Autodesk Fusion 360 part; units mm, degrees
sketch "Sketch1" plane through (0, 0, 0) normal (0, 0, 1) x (1, 0, 0) in component "Component"
  line L0 (-13, 0) -> (-13, 6.5)
  line L1 (-13, 0) -> (-13, -6.5)
  line L2 (-13, -6.5) -> (13, -6.5)
  line L3 (13, -6.5) -> (13, 6.5)
  line L4 (13, 6.5) -> (-13, 6.5)
  circle A0 centre (0, 0) radius 3
  line L5 (0, 0) -> (9.75, 0)
  line L6 (0, 0) -> (-9.75, 0)
  circle A1 centre (-9.75, 0) radius 3
  circle A2 centre (9.75, 0) radius 3
  line L7 (13, -6.5) -> (14, -6.5)
  line L8 (14, -6.5) -> (14, 6.5)
  line L9 (14, 6.5) -> (13, 6.5)
  line L10 (-13, 6.5) -> (-14, 6.5)
  line L11 (-14, 6.5) -> (-14, -6.5)
  line L12 (-14, -6.5) -> (-13, -6.5)
  dimension "d2" = 13
  dimension "d3" = 6.5
  dimension "d4" = 6.5
  dimension "d5" = 13
  dimension "d6" = 9.75
  dimension "d7" = 9.75
  dimension "d8" = 6
  dimension "d9" = 6
  dimension "d10" = 13
  dimension "d11" = 13
extrude "Extrude1" add sketch "Sketch1" along normal blind 2.5 in component "Component"
component "Component" placed x (1, 0, 0) y (0, 1, 0) z (0, 0, 1) at (0, 0, 0)
Work out the finished part from the listing and answer in its coordinate system (mm). Coordinates: 2 decimals unless noted, no trailing zeros. Write each loop counter-clockwise with the first axis right and the second up, starting at its lowest first coordinate (ties: lowest second). Pieces come first, ordered by that corner, then holes. Notation, with made-up numbers: (50.25, 1.5) - (98.25, 1.5) arc R24 ccw to (98.25, 20.5) - close; hole circle Ø5 at (74, 6). An arc over 180 degrees is marked (long way). One line per question, with ' | ' between items.
1) Find section A-A, the plane y = 0. Determine the outline of the cut face in (x, z), and give its area (3 significant figures).
Checks:
outline: (-14, 0) - (-12.75, 0) - (-12.75, 2.5) - (-14, 2.5) - close; (-6.75, 0) - (-3, 0) - (-3, 2.5) - (-6.75, 2.5) - close; (3, 0) - (6.75, 0) - (6.75, 2.5) - (3, 2.5) - close; (12.75, 0) - (14, 0) - (14, 2.5) - (12.75, 2.5) - close | area: 25.0 mm2
2) Consider probe 1 along X at (y, z) = (2, 0.85); probe 2 along Y at (x, z) = (-9.75, 0.6); probe 3 along X at (y, z) = (1.5, 1.3). Determine where each line is inside the solid, lowest interval first. Write a range as [from, to].
Checks:
probe 1: [-14, -11.99], [-7.51, -2.24], [2.24, 7.51], [11.99, 14] | probe 2: [-6.5, -3], [3, 6.5] | probe 3: [-14, -12.35], [-7.15, -2.6], [2.6, 7.15], [12.35, 14]
3) Find section C-C, the plane z = 1.05. Determine the outline of the cut face in (x, y), and give its area (3 significant figures).
Checks:
outline: (-14, -6.5) - (14, -6.5) - (14, 6.5) - (-14, 6.5) - close; hole circle Ø6 at (-9.75, 0); hole circle Ø6 at (0, 0); hole circle Ø6 at (9.75, 0) | area: 279 mm2
4) The mould has two halves that part along X. Classify faces 1 (the face through (14, 0, 1)), 2 (the face through (-12.131, 1.825, 1.232)), 3 (the face through (0, -6.5, 1)): +X half, -X half, draft (parallel to the pull), parting line (faces both ways), or undercut.
Checks:
face 1: +X half | face 2: undercut | face 3: draft
5) Find section D-D, the plane x = -11. Determine the outline of the cut face in (y, z), and give its area (3 significant figures).
Checks:
outline: (-6.5, 0) - (-2.73, 0) - (-2.73, 2.5) - (-6.5, 2.5) - close; (2.73, 0) - (6.5, 0) - (6.5, 2.5) - (2.73, 2.5) - close | area: 18.9 mm2
6) Find section B-B, the plane x = 0. Determine the outline of the cut face in (y, z).
Checks:
outline: (-6.5, 0) - (-3, 0) - (-3, 2.5) - (-6.5, 2.5) - close; (3, 0) - (6.5, 0) - (6.5, 2.5) - (3, 2.5) - close
